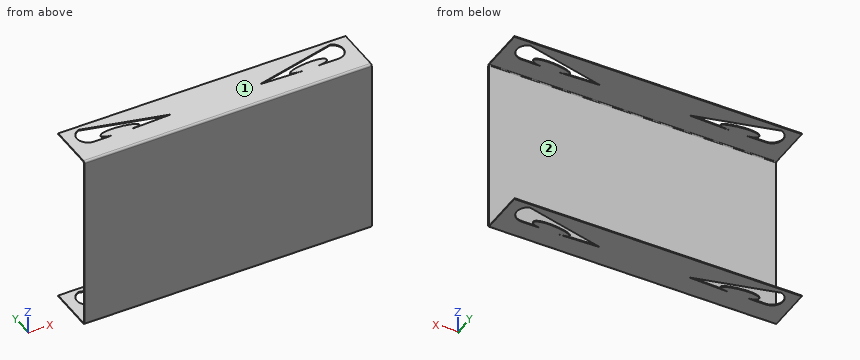
```python
from build123d import *

# Parameters (mm, degrees)
SKETCH1_W                      = 219
SKETCH1_H                      = 135
BASE_FLANGE1_DEPTH             = 0.7366
EDGE_FLANGE1_STRIP_W           = 4.4196
EDGE_FLANGE1_STRIP_H           = 0.7366
EDGE_FLANGE1_STRIP_CUT_DEPTH   = 219
EDGE_FLANGE1_STRIP_2_W         = 4.4196
EDGE_FLANGE1_STRIP_2_H         = 0.7366
EDGE_FLANGE1_STRIP_CUT_2_DEPTH = 219
EDGE_FLANGE1_DEPTH             = 219
EDGE_FLANGE1_BEND_DEPTH        = 219
CUT_EXTRUDE1_DEPTH             = 179.438180663


# Sheet-metal steps are written as plain solids
with BuildPart() as part:
    # Sketch1 → Base-Flange1 (new body)
    with BuildSketch(Plane(origin=(0, 0, 0), x_dir=(1, 0, 0), z_dir=(0, 1, 0))):
        Rectangle(SKETCH1_W, SKETCH1_H)
    extrude(amount=-BASE_FLANGE1_DEPTH)

    # Edge-Flange1 strip (across the edge) → Edge-Flange1 strip cut (cut)
    with BuildSketch(Plane(origin=(-109.5, 0, 67.5), x_dir=(0, 0, -1), z_dir=(1, 0, 0))):
        with Locations((-1.4732, -0.3683)):
            Rectangle(EDGE_FLANGE1_STRIP_W, EDGE_FLANGE1_STRIP_H)
    extrude(amount=EDGE_FLANGE1_STRIP_CUT_DEPTH, mode=Mode.SUBTRACT)

    # Edge-Flange1 strip 2 (across the edge) → Edge-Flange1 strip cut 2 (cut)
    with BuildSketch(Plane(origin=(109.5, 0, -67.5), x_dir=(0, 0, 1), z_dir=(-1, 0, 0))):
        with Locations((-1.4732, -0.3683)):
            Rectangle(EDGE_FLANGE1_STRIP_2_W, EDGE_FLANGE1_STRIP_2_H)
    extrude(amount=EDGE_FLANGE1_STRIP_CUT_2_DEPTH, mode=Mode.SUBTRACT)

    # Edge-Flange1 section (across the edge) → Edge-Flange1 (add)
    with BuildSketch(Plane(origin=(-109.5, 0, 67.5), x_dir=(0, 0, -1), z_dir=(1, 0, 0))):
        with BuildLine():
            Line((-0.7366, 0.7366), (-0.7366, 35))
            Line((-0.7366, 35), (0, 35))
            Line((0, 35), (0, 0.7366))
            ThreePointArc((0, 0.7366), (0.215745145, 0.215745145), (0.7366, 0))
            Line((0.7366, 0), (0.7366, -0.7366))
            ThreePointArc((0.7366, -0.7366), (-0.30510971, -0.30510971), (-0.7366, 0.7366))
        make_face()
    extrude(amount=EDGE_FLANGE1_DEPTH)

    # Edge-Flange1 section 2 (across the edge) → Edge-Flange1 bend (add)
    with BuildSketch(Plane(origin=(109.5, 0, -67.5), x_dir=(0, 0, 1), z_dir=(-1, 0, 0))):
        with BuildLine():
            Line((-0.7366, 0.7366), (-0.7366, 35))
            Line((-0.7366, 35), (0, 35))
            Line((0, 35), (0, 0.7366))
            ThreePointArc((0, 0.7366), (0.215745145, 0.215745145), (0.7366, 0))
            Line((0.7366, 0), (0.7366, -0.7366))
            ThreePointArc((0.7366, -0.7366), (-0.30510971, -0.30510971), (-0.7366, 0.7366))
        make_face()
    extrude(amount=EDGE_FLANGE1_BEND_DEPTH)

    # Sketch13 → Cut-Extrude1 (cut, through all)
    with BuildSketch(Plane.XY.offset(68.2366)):
        with BuildLine():
            Line((77.825189915, 15.538033098), (93.129236627, 15.538033098))
            ThreePointArc((93.129236627, 15.538033098), (101.370995393, 22.515880602), (95.848230578, 31.795751945))
            Line((95.848230578, 31.795751945), (33.918811085, 16.589807391))
            Line((33.918811085, 16.589807391), (66.285317903, 15.384418636))
            add(Edge.make_bspline(
                [(66.285317903, 15.384418636), (33.918811085, 16.589807391), (95.848230578, 31.795751945), (93.129236627, 15.538033098), (77.825189915, 15.538033098)],
                knots=[0, 0, 0, 0, 0, 1, 1, 1, 1, 1], degree=4))
        make_face()
        with BuildLine():
            Line((-95.848230578, 31.795751945), (-33.918811085, 16.589807391))
            Line((-33.918811085, 16.589807391), (-66.285317903, 15.384418636))
            add(Edge.make_bspline(
                [(-66.285317903, 15.384418636), (-33.918811085, 16.589807391), (-95.848230578, 31.795751945), (-93.129236627, 15.538033098), (-77.825189915, 15.538033098)],
                knots=[0, 0, 0, 0, 0, 1, 1, 1, 1, 1], degree=4))
            Line((-77.825189915, 15.538033098), (-93.129236627, 15.538033098))
            ThreePointArc((-93.129236627, 15.538033098), (-101.370995393, 22.515880602), (-95.848230578, 31.795751945))
        make_face()
    extrude(amount=-CUT_EXTRUDE1_DEPTH, mode=Mode.SUBTRACT)


solid = part.part
```
Build history of the part. All positions in model axes, mm. Face numbers are marked on the shaded views. A direction names the side the tool comes from. Give positions to 0.01 mm unless a question says otherwise; leave off trailing zeros. Loops run counter-clockwise (first coordinate to the right, second up) from the corner with the lowest first, then second, coordinate; pieces in that order, holes last.
1) Probe line 1 along Z through (x, y) = (-63, 7); line 2 along Y through (x, z) = (41, 42). List the from-to ranges inside material, lowest first.
Values follow:
line 1: z = -68.24 to -67.5, 67.5 to 68.24
line 2: y = -0.74 to 0
2) Band-saw the part on C-C on y = 26. List the corners of the cut face in (x, z).
Values follow:
outline: (-109.5, -68.24) - (-101.22, -68.24) - (-101.22, -67.5) - (-109.5, -67.5) - close; (-109.5, 67.5) - (-101.22, 67.5) - (-101.22, 68.24) - (-109.5, 68.24) - close; (-72.24, -68.24) - (72.24, -68.24) - (72.24, -67.5) - (-72.24, -67.5) - close; (-72.24, 67.5) - (72.24, 67.5) - (72.24, 68.24) - (-72.24, 68.24) - close; (101.22, -68.24) - (109.5, -68.24) - (109.5, -67.5) - (101.22, -67.5) - close; (101.22, 67.5) - (109.5, 67.5) - (109.5, 68.24) - (101.22, 68.24) - close
3) 3-axis set-ups, long thin cutter, end or side, ignore diameter. For the marked faces 1 and 2: which of +Z, -Z, +X, -X, +Y, -Y reach the whole face in a straight line?
Values follow:
face 1: +Z, +X, -X, +Y, -Y
face 2: +X, -X, +Y
4) Band-saw the part on A-A on y = 13. List the corners of the cut face in (x, z), then the cut area to 3 significant figures.
Values follow:
outline: (-109.5, -68.24) - (109.5, -68.24) - (109.5, -67.5) - (-109.5, -67.5) - close; (-109.5, 67.5) - (109.5, 67.5) - (109.5, 68.24) - (-109.5, 68.24) - close
area: 323 mm2
5) Band-saw the part on D-D on x = 43. List the corners of the cut face in (y, z).
Values follow:
outline: (-0.74, -66.76) arc R1.47 ccw to (0.74, -68.24) - (16.25, -68.24) - (16.25, -67.5) - (0.74, -67.5) arc R0.74 cw to (0, -66.76) - (0, 66.76) arc R0.74 cw to (0.74, 67.5) - (16.25, 67.5) - (16.25, 68.24) - (0.74, 68.24) arc R1.47 ccw to (-0.74, 66.76) - close; (18.82, -68.24) - (35, -68.24) - (35, -67.5) - (18.82, -67.5) - close; (18.82, 67.5) - (35, 67.5) - (35, 68.24) - (18.82, 68.24) - close
6) Drop flat-ended pins along their axis: P1, Ø8, axis at x = 25.5, z = -26.5, coming from the +Y side; P2, Ø8, axis at y = 7.5, z = 23, coming from the -X side. Give the stop position or say it passes through.
Values follow:
P1: stops at y = 0
P2: passes through
7) Band-saw the part on B-B on x = -11. List the corners of the cut face in (y, z).
Values follow:
outline: (-0.74, -66.76) arc R1.47 ccw to (0.74, -68.24) - (35, -68.24) - (35, -67.5) - (0.74, -67.5) arc R0.74 cw to (0, -66.76) - (0, 66.76) arc R0.74 cw to (0.74, 67.5) - (35, 67.5) - (35, 68.24) - (0.74, 68.24) arc R1.47 ccw to (-0.74, 66.76) - close
